```python
from build123d import *

# Parameters (mm, degrees)
F0_R     = 9.525
F1_DEPTH = 25.4
F3_DEPTH = 25.401
F4_DEPTH = 12.065
F6_DEPTH = 9.525


with BuildPart() as f1:
    # F0 (on Front) → F1 (new body)
    with BuildSketch(Plane.XZ):
        Circle(F0_R)
    extrude(amount=F1_DEPTH)

    # F2 (on Front) → F3 (cut, through all)
    with BuildSketch(Plane.XZ):
        with BuildLine():
            ThreePointArc((-4.7625, 0), (-3.367596, -3.367596), (0, -4.7625))
            ThreePointArc((0, -4.7625), (3.367596, -3.367596), (4.7625, 0))
            ThreePointArc((4.7625, 0), (3.367596, 3.367596), (0, 4.7625))
            ThreePointArc((0, 4.7625), (-3.367596, 3.367596), (-4.7625, 0))
        make_face()
    extrude(amount=F3_DEPTH, mode=Mode.SUBTRACT)

    # F2 (on Front) → F4 (cut)
    with BuildSketch(Plane.XZ):
        with BuildLine():
            Line((0, -4.7625), (4.7625, -4.7625))
            Line((4.7625, -4.7625), (4.7625, 0))
            ThreePointArc((4.7625, 0), (3.367596, -3.367596), (0, -4.7625))
        make_face()
        with BuildLine():
            Line((-4.7625, -4.7625), (0, -4.7625))
            ThreePointArc((0, -4.7625), (-3.367596, -3.367596), (-4.7625, 0))
            Line((-4.7625, 0), (-4.7625, -4.7625))
        make_face()
        with BuildLine():
            ThreePointArc((0, 4.7625), (3.367596, 3.367596), (4.7625, 0))
            Line((4.7625, 0), (4.7625, 4.7625))
            Line((4.7625, 4.7625), (0, 4.7625))
        make_face()
        with BuildLine():
            Line((-4.7625, 4.7625), (-4.7625, 0))
            ThreePointArc((-4.7625, 0), (-3.367596, 3.367596), (0, 4.7625))
            Line((0, 4.7625), (-4.7625, 4.7625))
        make_face()
    extrude(amount=F4_DEPTH, mode=Mode.SUBTRACT)

    # F5 (on face) → F6 (cut)
    with BuildSketch(Plane(origin=(0, 0, 0), x_dir=(-1, 0, 0), z_dir=(0, 1, 0))):
        Polygon((4.794214, -5.66426), (7.3025, 1.319781), (2.508286, 6.984041), (-4.794214, 5.66426), (-7.3025, -1.319781), (-2.508286, -6.984041), align=None)
    extrude(amount=-F6_DEPTH, mode=Mode.SUBTRACT)


solid = f1.part
```
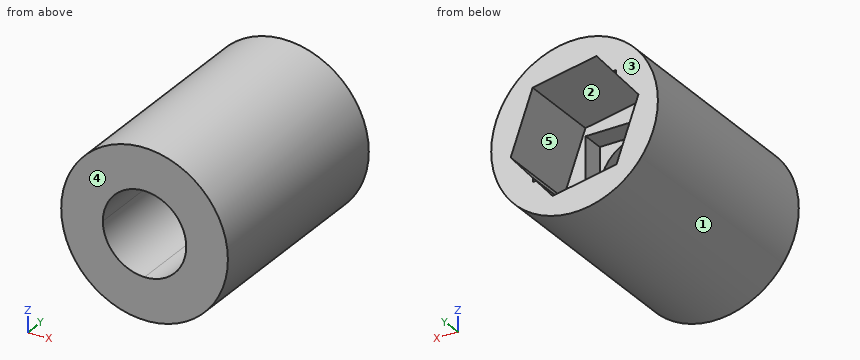
Build history of the part. All positions in model axes, mm. Face numbers are marked on the shaded views. A direction names the side the tool comes from. Give positions to 0.01 mm unless a question says otherwise; leave off trailing zeros. Use a Markdown table: item, result.
(1) Which spindle directions (+Z, -Z, +X, -X, +Y, -Y) get a long thin tool onto all of the face, cutting with end or side? Do the marked faces 4 and 5. Say none if no direction does.
Taken from the geometry:
| item | result |
|---|---|
| face 4 | +Z, -Z, +X, -X, -Y |
| face 5 | +Y |
(2) Wall check: line 1 along Z through (x, y) = (-2.5, -3.75); line 2 along Y through (x, z) = (-4.25, 4) (3 decimals); line 3 along Z through (x, y) = (-4, -10). Give the ranges that are in metal, low to high.
Taken from the geometry:
| item | result |
|---|---|
| line 1 | -9.19 to -6.08, 6.98 to 9.19 |
| line 2 | -25.4 to -12.065 |
| line 3 | -8.64 to -4.76, 4.76 to 8.64 |
(3) Pull direction X, two halves, no side cores. Call the marked faces 1, 2 and 3: +X half, -X half, draft (parallel to the pull), parting line (faces both ways), or undercut.
Taken from the geometry:
| item | result |
|---|---|
| face 1 | parting line |
| face 2 | undercut |
| face 3 | draft |
(4) Drop flat-ended pins along their axis: pin 1 Ø5 at (y, z) = (-8.5, 7) entering from -X (3 decimals); pin 2 Ø1.4 at (x, z) = (-3.5, 1.5) entering from +Y; pin 3 Ø4 at (x, z) = (1.5, 3.5) entering from +Y (3 decimals); pin 4 Ø1.5 at (y, z) = (-12.5, -7) entering from -X. Give the stop position or say it passes through.
Taken from the geometry:
| item | result |
|---|---|
| pin 1 | x = -8.395 |
| pin 2 | through |
| pin 3 | y = -9.525 |
| pin 4 | x = -7.19 |
